Can you work these out from the drawing? Everything is in mm from the part's minimum corner. A direction names the side the tool comes from. Round coordinates to 2 decimals unless told otherwise and drop trailing zeros. Order: outer loops, then holes, each group sorted by start corner. A loop starts at its lowest first (then second) coordinate and runs counter-clockwise, first axis right, second up. Notation, with made-up numbers: (81, 19.25) -> (101, 19.25) arc R21 cw to (101, 37.25) -> close; hole circle Ø7 at (11.25, -33). An arc over 180 degrees is marked (long way). One line per item, written item: value.
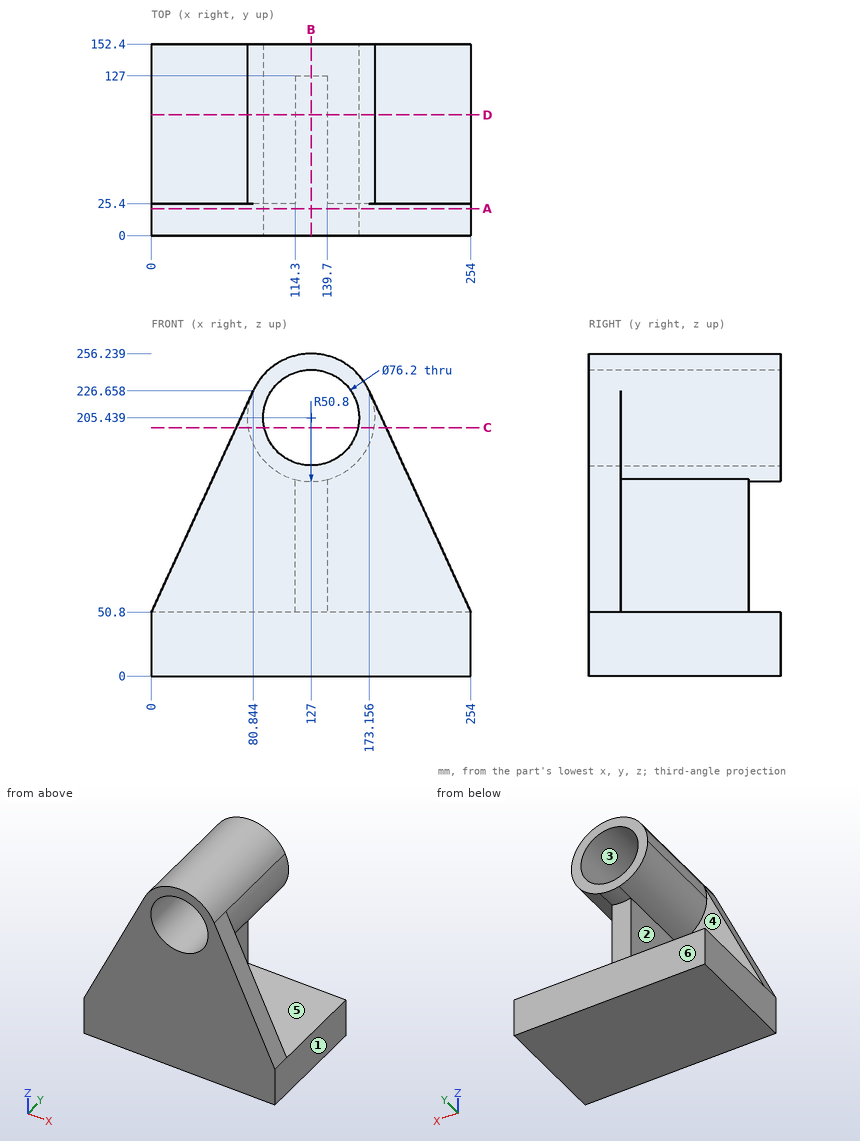
Q1. I want a section at D-D on y = 96. List the corners of the cut face in (x, z) for me, plus the area to 3 significant figures.
Answers below:
outline: (0, 0) -> (254, 0) -> (254, 50.8) -> (139.7, 50.8) -> (139.7, 156.25) arc R50.8 ccw (long way) to (114.3, 156.25) -> (114.3, 50.8) -> (0, 50.8) -> close; hole circle Ø76.2 at (127, 205.44)
area: 19,100 mm^2
Q2. I want a section at B-B on x = 127. List the corners of the cut face in (y, z) for me.
Answers below:
outline: (0, 0) -> (152.4, 0) -> (152.4, 50.8) -> (127, 50.8) -> (127, 154.64) -> (152.4, 154.64) -> (152.4, 167.34) -> (0, 167.34) -> close; (0, 243.54) -> (152.4, 243.54) -> (152.4, 256.24) -> (0, 256.24) -> close
Q3. We'd pull the mould along X, two halves only. Please class the marked faces 1, 2, 3 and 4: released by +X, released by -X, zero draft, split by the parting line, or undercut.
Answers below:
face 1: released by +X
face 2: released by -X
face 3: undercut
face 4: zero draft
Q4. Will these pins go through, and if not, where does the flat tip stop? pin 1 Ø8 at (x, y) = (219.5, 72.5) entering from +Z; pin 2 Ø10 at (y, z) = (131, 123) entering from -X.
Answers below:
pin 1: z = 50.8
pin 2: x = 114.3
Q5. I want a section at A-A on y = 21.5. List the corners of the cut face in (x, z) for me, plus the area to 3 significant figures.
Answers below:
outline: (0, 0) -> (254, 0) -> (254, 50.8) -> (173.16, 226.66) arc R50.8 ccw to (80.84, 226.66) -> (0, 50.8) -> close; hole circle Ø76.2 at (127, 205.44)
area: 40,800 mm^2
Q6. Please list where these lines run through material, in increasing order: line 1 along Z through (x, y) = (125, 11.5); line 2 along Z through (x, y) = (127, 69.5); line 3 along X through (y, z) = (50, 84).
Answers below:
line 1: 0 to 167.39, 243.49 to 256.2
line 2: 0 to 167.34, 243.54 to 256.24
line 3: 114.3 to 139.7
Q7. I want a section at C-C on z = 197.5. List the corners of the cut face in (x, y) for me (1 decimal).
Answers below:
outline: (67.4, 0) -> (89.7, 0) -> (89.7, 152.4) -> (76.8, 152.4) -> (76.8, 25.4) -> (67.4, 25.4) -> close; (164.3, 0) -> (186.6, 0) -> (186.6, 25.4) -> (177.2, 25.4) -> (177.2, 152.4) -> (164.3, 152.4) -> close
Q8. On a 3-axis mill with a long thin cutter (end or side, diameter ignored), from which of +Z, -Z, +X, -X, +Y, -Y can I reach the whole of each face in a straight line? I mean the marked faces 5 and 6. Say none if no direction works.
Answers below:
face 5: +Y
face 6: +Z, -Z, +X, -X, +Y
